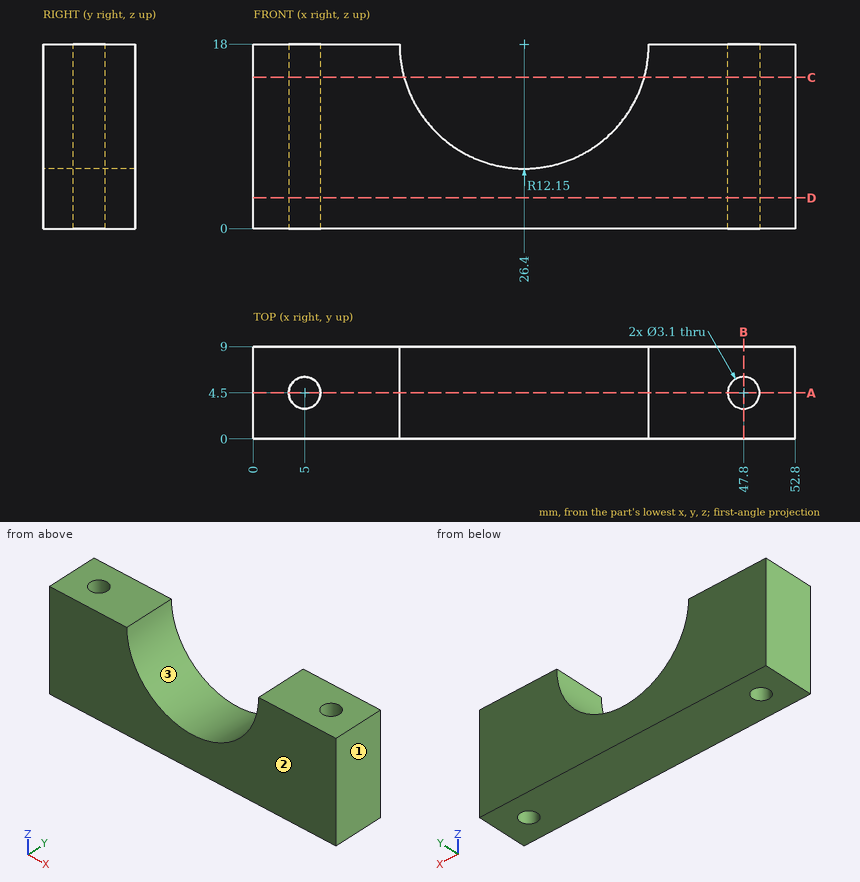
Verification items for this drawing (mm, ordinates from the low corner). Round coordinates to 2 decimals unless told otherwise and drop trailing zeros. Order: outer loops, then holes, each group sorted by start corner. A loop starts at its lowest first (then second) coordinate and runs counter-clockwise, first axis right, second up. Notation, with made-up numbers: (22.25, 38.25) - (40.25, 38.25) arc R14 cw to (40.25, 62.25) - close; hole circle Ø7 at (31, 69). An arc over 180 degrees is marked (long way). Answer as CSV lines item,"result". Start each with the question number.
1) Section check C-C (z = 14.75). Record the cut outline in (x, y), then the cut area to 3 significant figures.
2) Section check B-B (x = 47.8). Record the cut outline in (y, z).
3) Depth check by flat-ended pin: pin 1 (3.5 mm diameter, centred on x = 5, y = 4.5, fed in from -Z). Enter the tip coordinate at first touch or a pass-through.
4) Section check A-A (y = 4.5). Record the cut outline in (x, z).
5) Draft check along X on the marked faces 1, 2 and 3. Enter one of: +X half, -X half, draft (parallel to the pull), parting line (faces both ways), or undercut.
6) Section check D-D (z = 3). Record the cut outline in (x, y), then the cut area to 3 significant figures.
7) Scan lines: probe 1 along X at (y, z) = (3.75, 14); probe 2 along Y at (x, z) = (47.8, 5.5); probe 3 along X at (y, z) = (3.5, 11). Record each from-to range of solid material in increasing order.
Determined:
1,outline,"(0, 0) - (14.69, 0) - (14.69, 9) - (0, 9) - close; (38.11, 0) - (52.8, 0) - (52.8, 9) - (38.11, 9) - close; hole circle Ø3.1 at (5, 4.5); hole circle Ø3.1 at (47.8, 4.5)"
1,area,"249 mm^2"
2,outline,"(0, 0) - (2.95, 0) - (2.95, 18) - (0, 18) - close; (6.05, 0) - (9, 0) - (9, 18) - (6.05, 18) - close"
3,pin 1,"z = 0"
4,outline,"(0, 0) - (3.45, 0) - (3.45, 18) - (0, 18) - close; (6.55, 0) - (46.25, 0) - (46.25, 18) - (38.55, 18) arc R12.15 cw to (14.25, 18) - (6.55, 18) - close; (49.35, 0) - (52.8, 0) - (52.8, 18) - (49.35, 18) - close"
5,face 1,"+X half"
5,face 2,"draft"
5,face 3,"undercut"
6,outline,"(0, 0) - (52.8, 0) - (52.8, 9) - (0, 9) - close; hole circle Ø3.1 at (5, 4.5); hole circle Ø3.1 at (47.8, 4.5)"
6,area,"460 mm^2"
7,probe 1,"0 to 3.64, 6.36 to 14.93, 37.87 to 46.44, 49.16 to 52.8"
7,probe 2,"0 to 2.95, 6.05 to 9"
7,probe 3,"0 to 3.82, 6.18 to 16.47, 36.33 to 46.62, 48.98 to 52.8"
